Can you work these out from the model? Positions are in its coordinate system, mm. Face numbers are marked on the shaded views. A direction names the side the tool comes from. Give positions to 0.01 mm unless a question says otherwise; leave off trailing zeros. Write each loop counter-clockwise with the first axis right and the second up, starting at its lowest first coordinate (ties: lowest second). Pieces come first, ordered by that corner, then holes.
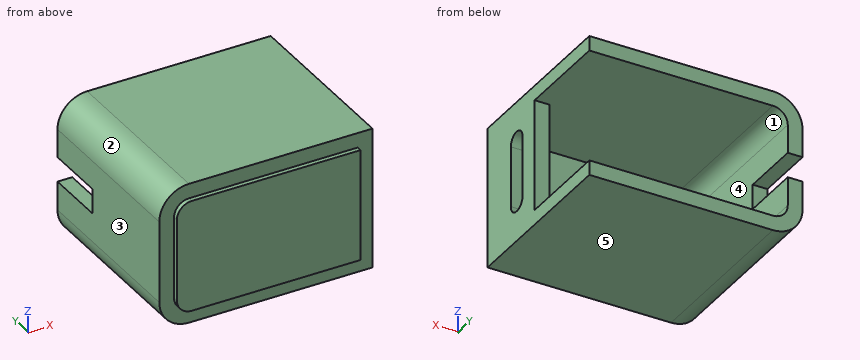
```python
from build123d import *

# Parameters (mm, degrees)
BOSS_EXTRUDE1_DEPTH = 33
SHELL2_T            = 3
SKETCH5_W           = 22.725
SKETCH5_H           = 33
CUT_EXTRUDE1_DEPTH  = 33
CUT_EXTRUDE3_START  = 20.6
SKETCH2_4_W         = 5.050381124
SKETCH2_4_H         = 5.05
CUT_EXTRUDE3_DEPTH  = 33
BOSS_EXTRUDE2_START = -4
BOSS_EXTRUDE2_DEPTH = 4
SKETCH6_W           = 3
SKETCH6_H           = 22.725
BOSS_EXTRUDE3_DEPTH = 13.67
CUT_EXTRUDE5_DEPTH  = 13.67


with BuildPart() as part:
    # Sketch2 → Boss-Extrude1 (new body)
    with BuildSketch(Plane(origin=(0, 0, 0), x_dir=(1, 0, 0), z_dir=(0, 1, 0))):
        with BuildLine():
            Line((21.210190562, 11.3625), (-13.129809438, 11.3625))
            ThreePointArc((-13.129809438, 11.3625), (-15.272342985, 10.475033547), (-16.159809438, 8.3325))
            Line((-16.159809438, 8.3325), (-16.159809438, -8.3325))
            ThreePointArc((-16.159809438, -8.3325), (-15.272342985, -10.475033547), (-13.129809438, -11.3625))
            Line((-13.129809438, -11.3625), (21.210190562, -11.3625))
            Line((21.210190562, -11.3625), (21.210190562, 11.3625))
        make_face()
    extrude(amount=BOSS_EXTRUDE1_DEPTH)

    # Shell2
    shell2_openings = [part.faces().sort_by_distance(p)[0] for p in [
        (2.609138826, 33, 0),
    ]]
    offset(amount=SHELL2_T, openings=shell2_openings, kind=Kind.INTERSECTION)

    # Sketch5 → Cut-Extrude1 (cut)
    with BuildSketch(Plane.ZY.offset(-21.210190562)):
        with Locations((0, 16.5)):
            Rectangle(SKETCH5_W, SKETCH5_H)
    extrude(amount=-CUT_EXTRUDE1_DEPTH, mode=Mode.SUBTRACT)

    # Sketch2_4 → Cut-Extrude3 (cut)
    with BuildSketch(Plane(origin=(0, 0, 0), x_dir=(1, 0, 0), z_dir=(0, 1, 0)).offset(CUT_EXTRUDE3_START)):
        with Locations((-18.685, -0.036435097)):
            Rectangle(SKETCH2_4_W, SKETCH2_4_H)
    extrude(amount=CUT_EXTRUDE3_DEPTH, mode=Mode.SUBTRACT)

    # Sketch2_6 → Boss-Extrude2 (add)
    with BuildSketch(Plane(origin=(0, 0, 0), x_dir=(1, 0, 0), z_dir=(0, 1, 0)).offset(BOSS_EXTRUDE2_START)):
        with BuildLine():
            Line((21.210190562, 11.3625), (-13.129809438, 11.3625))
            ThreePointArc((-13.129809438, 11.3625), (-15.272342985, 10.475033547), (-16.159809438, 8.3325))
            Line((-16.159809438, 8.3325), (-16.159809438, -8.3325))
            ThreePointArc((-16.159809438, -8.3325), (-15.272342985, -10.475033547), (-13.129809438, -11.3625))
            Line((-13.129809438, -11.3625), (21.210190562, -11.3625))
            Line((21.210190562, -11.3625), (21.210190562, 11.3625))
        make_face()
    extrude(amount=BOSS_EXTRUDE2_DEPTH)

    # Sketch6 → Boss-Extrude3 (add)
    with BuildSketch(Plane(origin=(0, 0, 0), x_dir=(1, 0, 0), z_dir=(0, 1, 0))):
        with Locations((22.710190562, 0)):
            Rectangle(SKETCH6_W, SKETCH6_H)
    extrude(amount=BOSS_EXTRUDE3_DEPTH)

    # Sketch7 → Cut-Extrude5 (cut)
    with BuildSketch(Plane(origin=(24.210190562, 0, 0), x_dir=(0, 0, -1), z_dir=(1, 0, 0))):
        with BuildLine():
            Line((-6.185942712, 9.395589147), (6.185942712, 9.395589147))
            ThreePointArc((6.185942712, 9.395589147), (8.247923616, 7.333608243), (6.185942712, 5.271627338))
            Line((6.185942712, 5.271627338), (-6.185942712, 5.271627338))
            ThreePointArc((-6.185942712, 5.271627338), (-8.247923616, 7.333608243), (-6.185942712, 9.395589147))
        make_face()
    extrude(amount=-CUT_EXTRUDE5_DEPTH, mode=Mode.SUBTRACT)


solid = part.part
```
1) Suppose I cut it at B-B on z = 0.25. Write out the boundary of the cut face in (x, y), plus the area to 3 significant figures.
Values follow:
outline: (-19.16, -3) - (-16.16, -3) - (-16.16, -4) - (21.21, -4) - (21.21, -3) - (24.21, -3) - (24.21, 5.27) - (21.21, 5.27) - (21.21, 0) - (-16.16, 0) - (-16.16, 20.6) - (-19.16, 20.6) - close; (21.21, 9.4) - (24.21, 9.4) - (24.21, 13.67) - (21.21, 13.67) - close
area: 258 mm2
2) For the marked faces 4 and 5, which set-ups out of +Z, -Z, +X, -X, +Y, -Y let a thin tool reach every point of the face, with its end or its side?
Values follow:
face 4: +Y
face 5: -Z, +X, -X, +Y, -Y
3) Suppose I cut it at A-A on y = 29. Write out the boundary of the cut face in (x, z), plus the area to 3 significant figures.
Values follow:
outline: (-19.16, -8.33) arc R6.03 ccw to (-13.13, -14.36) - (24.21, -14.36) - (24.21, -11.36) - (-13.13, -11.36) arc R3.03 cw to (-16.16, -8.33) - (-16.16, -2.49) - (-19.16, -2.49) - close; (-19.16, 2.56) - (-16.16, 2.56) - (-16.16, 8.33) arc R3.03 cw to (-13.13, 11.36) - (24.21, 11.36) - (24.21, 14.36) - (-13.13, 14.36) arc R6.03 ccw to (-19.16, 8.33) - close
area: 302 mm2
4) Suppose I cut it at D-D on y = 13. Write out the boundary of the cut face in (x, z).
Values follow:
outline: (-19.16, -8.33) arc R6.03 ccw to (-13.13, -14.36) - (24.21, -14.36) - (24.21, 14.36) - (-13.13, 14.36) arc R6.03 ccw to (-19.16, 8.33) - close; hole (-16.16, -8.33) arc R3.03 ccw to (-13.13, -11.36) - (21.21, -11.36) - (21.21, 11.36) - (-13.13, 11.36) arc R3.03 ccw to (-16.16, 8.33) - close
5) Please list where these lines run through material, in increasing order: L1, parallel to X at y = 12, z = 4.5; L2, parallel to Z at x = -12, y = 11.5; L3, parallel to Y at x = -9, z = -7.75.
Values follow:
L1: x = -19.16 to -16.16, 21.21 to 24.21
L2: z = -14.36 to -11.36, 11.36 to 14.36
L3: y = -4 to 0
6) If we mould it in two halves opening along Z, with no side actions, what happens to the marked faces 1, 2 and 3? For each: +Z half, -Z half, draft (parallel to the pull), parting line (faces both ways), or undercut.
Values follow:
face 1: undercut
face 2: +Z half
face 3: draft
7) For pin 1 Ø0.9 at (x, y) = (-17.5, 27) entering from +Z; pin 2 Ø12 at (y, z) = (27.5, 10.5) entering from -X; pin 3 Ø2.5 at (x, z) = (22, 1) entering from +Y; pin 4 Ø0.9 at (x, y) = (-18, 25) entering from -Z, each with a flat end and sliding along its axis, tell me the tip position at first contact or that it passes through.
Values follow:
pin 1: stops at z = 12.91
pin 2: stops at x = -19.16
pin 3: stops at y = 13.67
pin 4: stops at z = -12.43
8) Suppose I cut it at C-C on x = -7.5. Write out the boundary of the cut face in (y, z).
Values follow:
outline: (-4, -11.36) - (-3, -11.36) - (-3, -14.36) - (33, -14.36) - (33, -11.36) - (0, -11.36) - (0, 11.36) - (33, 11.36) - (33, 14.36) - (-3, 14.36) - (-3, 11.36) - (-4, 11.36) - close
